Model file for the job. Use its own axes, mm. A direction names the side the tool comes from. Coordinates: 2 decimals unless noted, no trailing zeros. Loops run counter-clockwise (first coordinate to the right, second up) from the corner with the lowest first, then second, coordinate; pieces in that order, holes last.
from build123d import *

# Parameters (mm, degrees)
F0_R     = 0.5
F1_DEPTH = 22.5
F2_W     = 1
F2_H     = 39
F2_W_2   = 0.5
F3_DEPTH = 25


with BuildPart() as f1:
    # F0 (on Front) → F1 (new body, symmetric)
    with BuildSketch(Plane.XZ):
        with BuildLine():
            ThreePointArc((-1, 1), (-2, 0), (-1, -1))
            Line((-1, -1), (1, -1))
            ThreePointArc((1, -1), (2, 0), (1, 1))
            Line((1, 1), (-1, 1))
        make_face()
        with Locations((-1, 0)):
            Circle(F0_R, mode=Mode.SUBTRACT)
        with Locations((1, 0)):
            Circle(F0_R, mode=Mode.SUBTRACT)
    extrude(amount=F1_DEPTH, both=True)

    # F2 (on face) → F3 (cut)
    with BuildSketch(Plane.XY.offset(1)):
        with Locations((1.5, 0)):
            Rectangle(F2_W, F2_H)
        with Locations((0.75, 0)):
            Rectangle(F2_W_2, F2_H)
        with Locations((-1.5, 0)):
            Rectangle(F2_W, F2_H)
        with Locations((-0.75, 0)):
            Rectangle(F2_W_2, F2_H)
    extrude(amount=-F3_DEPTH, mode=Mode.SUBTRACT)


solid = f1.part
Q1. Slice it at A-A (y = 9). List the corners of the cut face in (x, z), and give its area (3 significant figures).
Answers:
outline: (-0.5, -1) - (0.5, -1) - (0.5, 1) - (-0.5, 1) - close
area: 2.00 mm2
Q2. Mould opens along X. For faces 1 (the cylindrical face through (-2, 21, 0)), 2 (the flat face through (0, -22.5, 0)), 3 (the cylindrical face through (-1.4, 21, -0.3)) say: +X half, -X half, draft (parallel to the pull), parting line (faces both ways), or undercut.
Answers:
face 1: -X half
face 2: draft
face 3: undercut
Q3. Which spindle directions (+Z, -Z, +X, -X, +Y, -Y) get a long thin tool onto all of the face, cutting with end or side? Do faces 4 (the flat face through (0, 22.5, 0)), 5 (the flat face through (-0.5, 0, 0)), 6 (the flat face through (0.5, 0, 0)). Say none if no direction does.
Answers:
face 4: +Z, -Z, +X, -X, +Y
face 5: +Z, -Z, -X
face 6: +Z, -Z, +X
Q4. Flat gauge pins, fed straight in: P1, Ø1, axis at y = 2, z = -0.5, coming from the -X side; P2, Ø1, axis at y = 2, z = 0, coming from the +X side. Where does each tip first touch, or does it go through?
Answers:
P1: stops at x = -0.5
P2: stops at x = 0.5
Q5. Drill centre lines: line 1 (X direction, y = -21.8, z = 0); line 2 (Y direction, x = 1.55, z = 0.5); line 3 (Z direction, x = -1, y = -21.8). Where is each one in solid material? Low to high.
Answers:
line 1: x = -2 to -1.5, -0.5 to 0.5, 1.5 to 2
line 2: y = -22.5 to -19.5, 19.5 to 22.5
line 3: z = -1 to -0.5, 0.5 to 1
